from build123d import *

# Parameters (mm, degrees)
F0_W      = 63.5
F0_H      = 38.1
F1_DEPTH  = 6.35
F2_R      = 3.5505344057
F2_R_2    = 3.6174877647
F2_R_3    = 3.175
F3_DEPTH  = 25.4
F4_W      = 25.4
F4_H      = 12.7
F5_DEPTH  = 31.75
F6_R      = 6.35
F7_DEPTH  = 12.701
F8_R      = 9.525
F9_W      = 12.7
F9_H      = 9.7370275993
F10_DEPTH = 12.7
F12_DEPTH = 25.4


with BuildPart() as f1:
    # F0 (on Top) → F1 (new body)
    with BuildSketch(Plane.XY):
        with Locations((31.75, 19.05)):
            Rectangle(F0_W, F0_H)
    extrude(amount=F1_DEPTH)

    # F2 (on face) → F3 (cut)
    with BuildSketch(Plane.XY.offset(6.35)):
        with Locations((6.35, 6.35)):
            Circle(F2_R)
        with Locations((57.15, 6.35)):
            Circle(F2_R_2)
        with Locations((57.8531328631, 31.75)):
            Circle(F2_R_3)
    extrude(amount=-F3_DEPTH, mode=Mode.SUBTRACT)

    # F4 (on face) → F5 (join)
    with BuildSketch(Plane.XY.offset(6.35)):
        with Locations((12.7, 31.75)):
            Rectangle(F4_W, F4_H)
    extrude(amount=F5_DEPTH)

    # F6 (on face) → F7 (cut, through all)
    with BuildSketch(Plane.XZ.offset(-25.4)):
        with Locations((13.1049470376, 25.4064576301)):
            Circle(F6_R)
        with BuildLine():
            ThreePointArc((0, 25.8240551986), (2.9939347232, 33.8082957634), (10.3623142783, 38.1))
            Line((10.3623142783, 38.1), (0, 38.1))
            Line((0, 38.1), (0, 25.8240551986))
        make_face()
        with BuildLine():
            ThreePointArc((15.0376857217, 38.1), (22.4060652768, 33.8082957634), (25.4, 25.8240551986))
            Line((25.4, 25.8240551986), (25.4, 38.1))
            Line((25.4, 38.1), (15.0376857217, 38.1))
        make_face()
    extrude(amount=-F7_DEPTH, mode=Mode.SUBTRACT)

    # F8
    f8_edges = [f1.edges().sort_by_distance(p)[0] for p in [
        (0, 0, 3.175),
        (63.5, 0, 3.175),
    ]]
    fillet(f8_edges, radius=F8_R)

    # F9 (on face) → F10 (join)
    with BuildSketch(Plane.YZ.offset(25.4)):
        with Locations((31.75, 11.2185137997)):
            Rectangle(F9_W, F9_H)
    extrude(amount=F10_DEPTH)

    # F11 (on face) → F12 (cut)
    with BuildSketch(Plane.XZ.offset(-25.4)):
        with BuildLine():
            ThreePointArc((34.7881134803, 11.0440567401), (30.0940567401, 15.7381134803), (25.4, 11.0440567401))
            ThreePointArc((25.4, 11.0440567401), (26.7748573879, 7.7248573879), (30.0940567401, 6.35))
            ThreePointArc((30.0940567401, 6.35), (33.4132560924, 7.7248573879), (34.7881134803, 11.0440567401))
        make_face()
        with BuildLine():
            Line((38.1, 16.0870275993), (25.4, 16.0870275993))
            Line((25.4, 16.0870275993), (25.4, 11.0440567401))
            ThreePointArc((25.4, 11.0440567401), (30.0940567401, 15.7381134803), (34.7881134803, 11.0440567401))
            ThreePointArc((34.7881134803, 11.0440567401), (33.4132560924, 7.7248573879), (30.0940567401, 6.35))
            Line((30.0940567401, 6.35), (38.1, 6.35))
            Line((38.1, 6.35), (38.1, 16.0870275993))
        make_face()
    extrude(amount=-F12_DEPTH, mode=Mode.SUBTRACT)


solid = f1.part
Geometry: final body of the model. Coordinates: model frame, mm. A direction names the side the tool comes from. Round coordinates to 2 decimals unless told otherwise and drop trailing zeros. Loops run counter-clockwise (first coordinate to the right, second up) from the corner with the lowest first, then second, coordinate; pieces in that order, holes last. Notation, with made-up numbers: (0.25, -17) - (13.25, -17) arc R19 cw to (13.25, 7) - close; hole circle Ø1 at (46, 35). An arc over 180 degrees is marked (long way). Write each question's results on one line, items separated by ' | '. Start each with the question number.
1) Cut plane D-D on x = 56.5. Return loops of the section in (y, z), then the cut area to 3 significant figures.
2) Line query: probe 1 along Y at (x, z) = (57.15, 4.5); probe 2 along Z at (x, y) = (16.5, 25). Output: solid intervals per line, ascending. Write a range as [from, to].
3) Access query for faces 1 (the face through (15, 25.4, 18)), 2 (the face through (24, 38.1, 15)), 3 (the face through (25.4, 32, 18)). Directions: +Z, -Z, +X, -X, +Y, -Y. A direction counts if a zero-diameter tool reaches every point of the face in a straight line with its end or side. Return the directions, or none.
4) Cut plane B-B on x = 17.5. Return loops of the section in (y, z).
5) Cut plane A-A on y = 31.75. Return loops of the section in (x, z).
6) First-contact query: P1, Ø3, axis at x = 50, y = 12.5, coming from the +Z side; P2, Ø15, axis at x = 11, z = 30, coming from the -Y side; P3, Ø14, axis at y = 30, z = 15.5, coming from the +X side. Flat tips, straight axial feed; report the tip coordinate or a pass-through.
7) Mould query, pull axis X, two halves, no side actions, for faces 4 (the face through (60.64, 2.72, 3.22)), 5 (the face through (2.72, 2.86, 3.22)), 6 (the face through (53.536, 6.509, 3.219)), 7 (the face through (31, 19, 6.35)). Classes: released by +X, released by -X, zero draft, split by the parting line, or undercut.
8) Cut plane C-C on y = 5.5. Return loops of the section in (x, z), then the cut area to 3 significant figures.
Verdict:
1) outline: (0.34, 0) - (2.79, 0) - (2.79, 6.35) - (0.34, 6.35) - close; (9.91, 0) - (28.88, 0) - (28.88, 6.35) - (9.91, 6.35) - close; (34.62, 0) - (38.1, 0) - (38.1, 6.35) - (34.62, 6.35) - close | area: 158 mm2
2) probe 1: y = [0.54, 2.73], [9.97, 28.65], [34.85, 38.1] | probe 2: z = [0, 6.35]
3) face 1: +Z, +X, -X, -Y | face 2: +Z, -Z, +X, -X, +Y | face 3: +Z, +X, +Y, -Y
4) outline: (0, 0) - (38.1, 0) - (38.1, 20.82) - (25.4, 20.82) - (25.4, 6.35) - (0, 6.35) - close; (25.4, 29.99) - (38.1, 29.99) - (38.1, 37.38) - (25.4, 37.38) - close
5) outline: (0, 0) - (54.68, 0) - (54.68, 6.35) - (30.09, 6.35) arc R4.69 cw to (25.4, 11.04) - (25.4, 25.82) arc R12.7 ccw to (15.04, 38.1) - (10.36, 38.1) arc R12.7 ccw to (0, 25.82) - close; (61.03, 0) - (63.5, 0) - (63.5, 6.35) - (61.03, 6.35) - close; hole circle Ø12.7 at (13.1, 25.41)
6) P1: stops at z = 6.35 | P2: stops at y = 25.4 | P3: stops at x = 26.15
7) face 4: released by +X | face 5: released by -X | face 6: undercut | face 7: zero draft
8) outline: (0.89, 0) - (2.9, 0) - (2.9, 6.35) - (0.89, 6.35) - close; (9.8, 0) - (53.63, 0) - (53.63, 6.35) - (9.8, 6.35) - close; (60.67, 0) - (62.61, 0) - (62.61, 6.35) - (60.67, 6.35) - close | area: 303 mm2
